from build123d import *

# Parameters (mm, degrees)
SKETCH_1_R          = 2.2
EXTRUDE_1_DEPTH     = 24
CUT_EXTRUDE_START   = -4
CUT_EXTRUDE_1_DEPTH = 17
FILLET_1_R          = 1


with BuildPart() as part:
    # 草图1 → 凸台-拉伸1 (new body)
    with BuildSketch(Plane.XY):
        with BuildLine():
            ThreePointArc((-71.830585516, -142.550559143), (-72.368769012, -144.398530389), (-71.098720838, -145.844772706))
            Line((-71.098720838, -145.844772706), (5.461936424, -145.844772706))
            ThreePointArc((5.461936424, -145.844772706), (6.731984597, -144.398530389), (6.193801102, -142.550559143))
            Line((6.193801102, -142.550559143), (-28.806198899, -107.550559143))
            ThreePointArc((-28.806198899, -107.550559143), (-29.455045597, -107.11701364), (-30.220412461, -106.964772705))
            Line((-30.220412461, -106.964772705), (-35.416371953, -106.964772705))
            ThreePointArc((-35.416371953, -106.964772705), (-36.181738818, -107.11701364), (-36.830585516, -107.550559143))
            Line((-36.830585516, -107.550559143), (-71.830585516, -142.550559143))
        make_face()
        with Locations((-64.818392207, -140.964772706)):
            Circle(SKETCH_1_R, mode=Mode.SUBTRACT)
        with Locations((-0.818392207, -140.964772706)):
            Circle(SKETCH_1_R, mode=Mode.SUBTRACT)
        with Locations((-32.818392207, -110.964772705)):
            Circle(SKETCH_1_R, mode=Mode.SUBTRACT)
    extrude(amount=EXTRUDE_1_DEPTH)

    # 草图2 → 切除-拉伸1 (cut)
    with BuildSketch(Plane.XY.offset(24).offset(CUT_EXTRUDE_START)):
        with BuildLine():
            Line((-40.067129549, -110.787103176), (-36.353926113, -114.500306611))
            ThreePointArc((-36.353926113, -114.500306611), (-32.818392207, -115.964772705), (-29.282858301, -114.500306611))
            Line((-29.282858301, -114.500306611), (-25.569654866, -110.787103176))
            Line((-25.569654866, -110.787103176), (-32.818392207, -103.538365834))
            Line((-32.818392207, -103.538365834), (-40.067129549, -110.787103176))
        make_face()
        with BuildLine():
            Line((-63.996061737, -134.716035364), (-61.282858301, -137.4292388))
            ThreePointArc((-61.282858301, -137.4292388), (-60.198994545, -139.051355544), (-59.818392207, -140.964772706))
            Line((-59.818392207, -140.964772706), (-59.818392207, -145.844772706))
            Line((-59.818392207, -145.844772706), (-75.124799079, -145.844772706))
            Line((-75.124799079, -145.844772706), (-63.996061737, -134.716035364))
        make_face()
        with BuildLine():
            Line((9.488014664, -145.844772706), (-5.818392207, -145.844772706))
            Line((-5.818392207, -145.844772706), (-5.818392207, -140.964772706))
            ThreePointArc((-5.818392207, -140.964772706), (-5.43778987, -139.051355544), (-4.353926113, -137.4292388))
            Line((-4.353926113, -137.4292388), (-1.640722678, -134.716035364))
            Line((-1.640722678, -134.716035364), (9.488014664, -145.844772706))
        make_face()
    extrude(amount=-CUT_EXTRUDE_1_DEPTH, mode=Mode.SUBTRACT)

    # 圆角1
    fillet_1_edges = [part.edges().sort_by_distance(p)[0] for p in [
        (-59.818392207, -145.844772706, 11.5),
        (-63.996061737, -134.716035364, 11.5),
        (-1.640722678, -134.716035364, 11.5),
        (-5.818392207, -145.844772706, 11.5),
        (-40.067129549, -110.787103176, 11.5),
        (-25.569654866, -110.787103176, 11.5),
    ]]
    fillet(fillet_1_edges, radius=FILLET_1_R)


solid = part.part
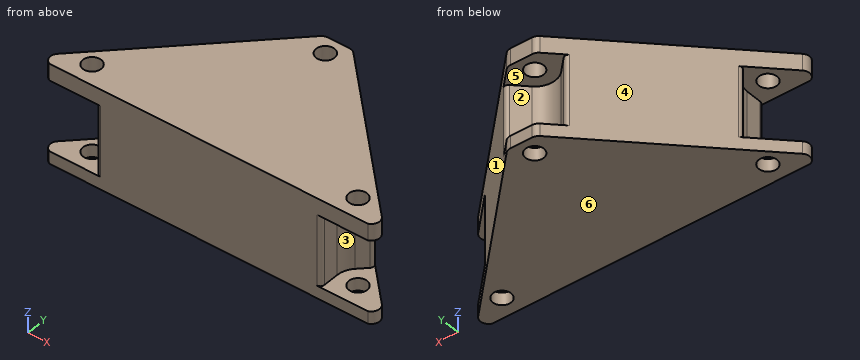
Design review of the part built by this model. Coordinates are the model's own, in mm. Face numbers are marked on the shaded views. A direction names the side the tool comes from. Coordinates: 2 decimals unless noted, no trailing zeros. Order: outer loops, then holes, each group sorted by start corner. A loop starts at its lowest first (then second) coordinate and runs counter-clockwise, first axis right, second up.
Item 1: Take a section at A-A, the plane y = -139.5. Write out the cut boundary in (x, z), then the cut area to 3 significant figures.
Item 2: For line 1 (X direction, y = -142, z = 21.5); line 2 (X direction, y = -115.5, z = 15.25); line 3 (X direction, y = -113, z = 12.75), list the stretches that pass through material, from the lowest coordinate up.
Item 3: For pin 1 Ø10 at (y, z) = (-124.5, 2.5) entering from -X; pin 2 Ø6 at (y, z) = (-139.5, 13) entering from -X; pin 3 Ø10 at (x, z) = (-31.5, 13.5) entering from +Y; pin 4 Ø2.5 at (x, y) = (-32.82, -110.96) entering from +Z, all flat-tipped, find the tip position at first contact; note any pin that passes through.
Item 4: Take a section at B-B, the plane z = 8. Write out the cut boundary in (x, y), then the cut area to 3 significant figures.
Item 5: For the marked faces 1, 2 and 3, list the 3-axis set-ups (+Z, -Z, +X, -X, +Y, -Y) from which the entire face can be reached by the end or side of a thin tool; tool diameter is ignored.
Item 6: Take a section at D-D, the plane y = -122. Write out the cut boundary in (x, z), then the cut area to 3 significant figures.
Item 7: Take a section at C-C, the plane x = -57.5. Write out the cut boundary in (y, z).
Item 8: The part is to be moulded in two halves that separate along Z. For the marked faces 4, 5 and 6, say which applies: pulls with the +Z half, pulls with the -Z half, needs draft (parallel to the pull), parting line crosses it, or undercut.
The answers:
1. outline: (-68.78, 0) - (-66.46, 0) - (-66.46, 3) - (-68.78, 3) - close; (-68.78, 20) - (-66.46, 20) - (-66.46, 24) - (-68.78, 24) - close; (-63.18, 0) - (-2.46, 0) - (-2.46, 3) - (-5.6, 3) - (-5.6, 20) - (-2.46, 20) - (-2.46, 24) - (-63.18, 24) - (-63.18, 20) - (-60.04, 20) - (-60.04, 3) - (-63.18, 3) - close; (0.82, 0) - (3.14, 0) - (3.14, 3) - (0.82, 3) - close; (0.82, 20) - (3.14, 20) - (3.14, 24) - (0.82, 24) - close
1. area: 1,380 mm2
2. line 1: x = -71.28 to -66.76, -62.88 to -2.76, 1.12 to 5.64
2. line 2: x = -44.78 to -34.92, -30.71 to -20.86
2. line 3: x = -42.28 to -37.85, -27.78 to -23.36
3. pin 1: stops at x = -58.78
3. pin 2: stops at x = -62.21
3. pin 3: stops at y = -111.72
3. pin 4: passes through
4. outline: (-63.29, -135.42) - (-61.28, -137.43) arc R5 cw to (-59.82, -140.96) - (-59.82, -144.84) arc R1 ccw to (-58.82, -145.84) - (-6.82, -145.84) arc R1 ccw to (-5.82, -144.84) - (-5.82, -140.96) arc R5 cw to (-4.35, -137.43) - (-2.35, -135.42) arc R1 ccw to (-2.35, -134.01) - (-24.86, -111.49) arc R1 ccw to (-26.28, -111.49) - (-29.28, -114.5) arc R5 cw to (-36.35, -114.5) - (-39.36, -111.49) arc R1 ccw to (-40.77, -111.49) - (-63.29, -134.01) arc R1 ccw to start
4. area: 1,490 mm2
5. face 1: +Z, -Z, +X, +Y
5. face 2: +Y
5. face 3: +X, -Y
6. outline: (-51.28, 0) - (-14.36, 0) - (-14.36, 24) - (-51.28, 24) - close
6. area: 886 mm2
7. outline: (-145.84, 0) - (-128.22, 0) - (-128.22, 24) - (-145.84, 24) - close
8. face 4: needs draft
8. face 5: undercut
8. face 6: pulls with the -Z half
